```python
from build123d import *

# Parameters (mm, degrees)
F0_W     = 29
F0_H     = 24
F0_W_2   = 25
F0_H_2   = 20
F1_DEPTH = 38.1
F2_DEPTH = 2
F3_W     = 20
F3_H     = 38.1
F4_DEPTH = 29.001
F6_DEPTH = 40.101


with BuildPart() as f1:
    # F0 (on Top) → F1 (new body)
    with BuildSketch(Plane.XY):
        Rectangle(F0_W, F0_H)
        Rectangle(F0_W_2, F0_H_2, mode=Mode.SUBTRACT)
    extrude(amount=F1_DEPTH)

    # F0 (on Top) → F2 (join)
    with BuildSketch(Plane.XY):
        Rectangle(F0_W, F0_H)
        Rectangle(F0_W_2, F0_H_2, mode=Mode.SUBTRACT)
        Rectangle(F0_W_2, F0_H_2)
    extrude(amount=-F2_DEPTH)

    # F3 (on face) → F4 (cut, through all)
    with BuildSketch(Plane(origin=(-14.5, 0, 0), x_dir=(0, -1, 0), z_dir=(-1, 0, 0))):
        with Locations((0, 19.05)):
            Rectangle(F3_W, F3_H)
    extrude(amount=-F4_DEPTH, mode=Mode.SUBTRACT)

    # F5 (on face) → F6 (cut, through all)
    with BuildSketch(Plane(origin=(0, 0, -2), x_dir=(1, 0, 0), z_dir=(0, 0, -1))):
        Polygon((-12.5, 10), (-12.5, 12), (-14.5, 12), (-14.5, -12), (-12.5, -12), (-12.5, -10), align=None)
        Polygon((14.5, -12), (14.5, 12), (12.5, 12), (12.5, 10), (12.5, -10), (12.5, -12), align=None)
    extrude(amount=-F6_DEPTH, mode=Mode.SUBTRACT)


solid = f1.part
```
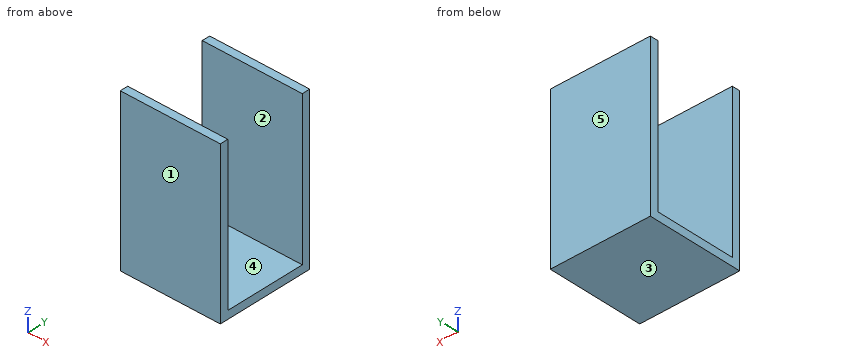
Source: CAD feature listing. Evaluate the final solid. Frame: model axes, mm. Face numbers are marked on the shaded views. A direction names the side the tool comes from. Coordinates: 2 decimals unless noted, no trailing zeros. Loops run counter-clockwise (first coordinate to the right, second up) from the corner with the lowest first, then second, coordinate; pieces in that order, holes last. Notation, with made-up numbers: M -21,29 L 25,29 A35 cw 25,62 Z; hole C 77,88.5 d10. An arc over 180 degrees is marked long. Use a Markdown table: item, result. Add a question column.
Q1. Section query B-B, the plane x = -4. Return loops of the section in (y, z).
Q2. Draft query along Y for the marked faces 3, 4 and 5. Return one class per face: pulls with the +Y half, pulls with the -Y half, needs draft (parallel to the pull), parting line crosses it, or undercut.
Q3. Access query for the marked faces 1 and 2. Directions: +Z, -Z, +X, -X, +Y, -Y. A direction counts if a zero-diameter tool reaches every point of the face in a straight line with its end or side. Return the directions, or none.
Q4. Material intervals for L1, parallel to Y at x = 2.75, z = 18.5; L2, parallel to Z at x = 4.5, y = 5.5, sorted ascending.
Q5. First-contact query: pin 1 (1.5 mm diameter, centred on x = -6.5, y = 8.5, fed in from +Z). Flat tip, straight axial feed; report the tip coordinate or a pass-through.
Q6. Section query C-C, the plane y = -4.75. Return loops of the section in (x, z).
Q7. Section query A-A, the plane z = 25.5. Return loops of the section in (x, y), and give its area (3 significant figures).
Result:
| question | item | result |
|---|---|---|
| 1 | outline | M -12,-2 L 12,-2 L 12,38.1 L 10,38.1 L 10,0 L -10,0 L -10,38.1 L -12,38.1 Z |
| 2 | face 3 | needs draft |
| 2 | face 4 | undercut |
| 2 | face 5 | pulls with the +Y half |
| 3 | face 1 | +Z, -Z, +X, -X, -Y |
| 3 | face 2 | +Z, +X, -X |
| 4 | L1 | y = -12 to -10, 10 to 12 |
| 4 | L2 | z = -2 to 0 |
| 5 | pin 1 | stops at z = 0 |
| 6 | outline | M -12.5,-2 L 12.5,-2 L 12.5,0 L -12.5,0 Z |
| 7 | outline | M -12.5,-12 L 12.5,-12 L 12.5,-10 L -12.5,-10 Z; M -12.5,10 L 12.5,10 L 12.5,12 L -12.5,12 Z |
| 7 | area | 100 mm2 |
